Input: part model. Units: mm. Frame: model coordinates. A direction names the side the tool comes from. Coordinates: 2 decimals unless noted, no trailing zeros. Order: outer loops, then holes, each group sorted by start corner. A loop starts at its lowest first (then second) coordinate and runs counter-clockwise, first axis right, second up. Notation, with made-up numbers: (-22, 37) -> (18, 37) arc R14 cw to (18, 63) -> close; hole circle Ø4 at (56.25, 19). An arc over 180 degrees is marked (long way). One line per item, written item: value. Start each with the question number.
from build123d import *

# Parameters (mm, degrees)
F0_R     = 15.24
F1_DEPTH = 31.75
F2_R     = 3.81
F3_R     = 2.413
F4_DEPTH = 101.6


with BuildPart() as f1:
    # F0 (on Front) → F1 (new body)
    with BuildSketch(Plane.XZ):
        Circle(F0_R)
    extrude(amount=F1_DEPTH)

    # F2
    f2_edges = [f1.edges().sort_by_distance(p)[0] for p in [
        (-15.24, -31.75, 0),
        (-15.24, 0, 0),
    ]]
    fillet(f2_edges, radius=F2_R)

    # F3 (on face) → F4 (join)
    with BuildSketch(Plane(origin=(0, 0, 0), x_dir=(-1, 0, 0), z_dir=(0, 1, 0))):
        Circle(F3_R)
    extrude(amount=F4_DEPTH)


solid = f1.part
1) Section query D-D, the plane y = -18. Return the cut outline in (x, z), plus the area to 3 significant figures.
2) Section query B-B, the plane z = 0. Return the cut outline in (x, y).
3) Access query for faces 1 (the cylindrical face through (1.915, 50.089, -1.468)), 2 (the cylindrical face through (-3.3, -15.71, -14.88)). Directions: +Z, -Z, +X, -X, +Y, -Y. A direction counts if a zero-diameter tool reaches every point of the face in a straight line with its end or side. Return the directions, or none.
4) Pin query (flat end, axial travel): pin 1 Ø5 at (x, y) = (-3.5, -3.5) entering from -Z; pin 2 Ø3 at (x, z) = (-3.5, -3) entering from +Y; pin 3 Ø4 at (y, z) = (-4.5, 6.5) entering from -X; pin 4 Ø7 at (x, z) = (5.5, -2) entering from +Y. Return the tip coordinate at first contact, or that it passes through.
5) Section query C-C, the plane y = 50. Return the cut outline in (x, z), plus the area to 3 significant figures.
6) Ray query, line 1 along Y through (x, z) = (-2, -6.5); line 2 along Y through (x, z) = (7, 13); line 3 along Z through (x, y) = (-1.5, -7.5). Return the intervals inside material, ascending. Write a range as from..to.
7) Section query A-A, the plane x = 0. Return the cut outline in (y, z), plus the area to 3 significant figures.
Entries:
1. outline: circle Ø30.48 at (0, 0)
1. area: 730 mm2
2. outline: (-15.24, -27.94) arc R3.81 ccw to (-11.43, -31.75) -> (11.43, -31.75) arc R3.81 ccw to (15.24, -27.94) -> (15.24, -3.81) arc R3.81 ccw to (11.43, 0) -> (2.41, 0) -> (2.41, 101.6) -> (-2.41, 101.6) -> (-2.41, 0) -> (-11.43, 0) arc R3.81 ccw to (-15.24, -3.81) -> close
3. face 1: +Y
3. face 2: +Y, -Y
4. pin 1: stops at z = -15.21
4. pin 2: stops at y = 0
4. pin 3: stops at x = -14.56
4. pin 4: stops at y = 101.6
5. outline: circle Ø4.83 at (0, 0)
5. area: 18.3 mm2
6. line 1: y = -31.75..0
6. line 2: y = -29.78..-1.97
6. line 3: z = -15.17..15.17
7. outline: (-31.75, -11.43) arc R3.81 ccw to (-27.94, -15.24) -> (-3.81, -15.24) arc R3.81 ccw to (0, -11.43) -> (0, -2.41) -> (101.6, -2.41) -> (101.6, 2.41) -> (0, 2.41) -> (0, 11.43) arc R3.81 ccw to (-3.81, 15.24) -> (-27.94, 15.24) arc R3.81 ccw to (-31.75, 11.43) -> close
7. area: 1,450 mm2
